```python
from build123d import *

# Parameters (mm, degrees)
SKETCH1_W           = 76.2
SKETCH1_H           = 50.8
SKETCH1_R           = 6.35
BOSS_EXTRUDE1_DEPTH = 3.175
BOSS_EXTRUDE2_DEPTH = 38.1
FILLET1_R           = 3.175
SKETCH3_2_R         = 4.7625
BOSS_EXTRUDE3_DEPTH = 31.75


with BuildPart() as part:
    # Sketch1 → Boss-Extrude1 (new body)
    with BuildSketch(Plane.XY):
        Rectangle(SKETCH1_W, SKETCH1_H)
        with Locations((-25.4, 0)):
            Circle(SKETCH1_R, mode=Mode.SUBTRACT)
        with Locations((25.4, 0)):
            Circle(SKETCH1_R, mode=Mode.SUBTRACT)
    extrude(amount=BOSS_EXTRUDE1_DEPTH)

    # Sketch2 → Boss-Extrude2 (add)
    with BuildSketch(Plane(origin=(0, 0, 0), x_dir=(0, 0, -1), z_dir=(1, 0, 0))):
        with BuildLine():
            Line((0, 38.1), (0, 25.4))
            Line((0, 25.4), (-3.175, 25.4))
            Line((-3.175, 25.4), (-3.175, 31.000484171))
            ThreePointArc((-3.175, 31.000484171), (-18.2200956, 41.988564967), (0, 38.1))
        make_face()
    extrude(amount=-BOSS_EXTRUDE2_DEPTH)

    # Fillet1
    fillet1_edges = [part.edges().sort_by_distance(p)[0] for p in [
        (-19.05, 31.000484171, 3.175),
    ]]
    fillet(fillet1_edges, radius=FILLET1_R)

    # Sketch3<2> → Boss-Extrude3 (add)
    with BuildSketch(Plane(origin=(0, 0, 0), x_dir=(0, 0, -1), z_dir=(1, 0, 0))):
        with Locations((-9.525, 38.1)):
            Circle(SKETCH3_2_R)
    extrude(amount=BOSS_EXTRUDE3_DEPTH)


solid = part.part
```
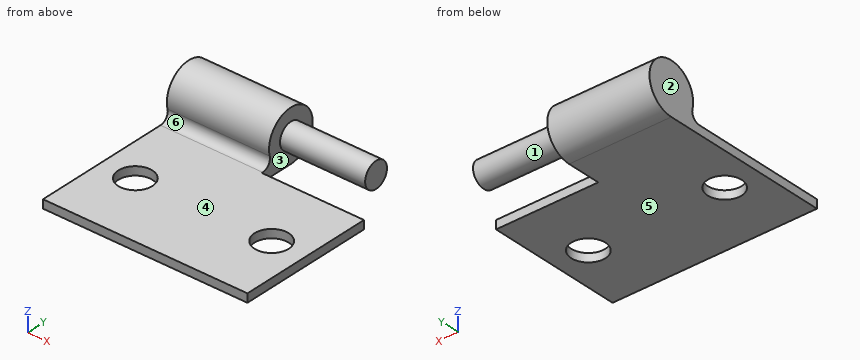
Verification items for the finished model (mm, model axes). Face numbers are marked on the shaded views. A direction names the side the tool comes from. Round coordinates to 2 decimals unless told otherwise and drop trailing zeros. Order: outer loops, then holes, each group sorted by start corner. A loop starts at its lowest first (then second) coordinate and runs counter-clockwise, first axis right, second up. Notation, with made-up numbers: (61, -9) -> (77, -9) arc R34 ccw to (77, 27) -> close; hole circle Ø2 at (-15.5, 60.5). An arc over 180 degrees is marked (long way). Put each result on its own line as item: value. Start each with the question number.
(1) Section check C-C (z = 12.5). Enter the section's corners in (x, y).
(2) Section check D-D (z = 2). Enter the section's corners in (x, y), then the cut area to 3 significant figures.
(3) Section check A-A (y = 0). Enter the section's corners in (x, z) (3 decimals).
(4) Depth check by flat-ended pin: pin 1 Ø4 at (x, z) = (-22.5, 9) entering from -Y (3 decimals); pin 2 Ø10 at (x, z) = (5.5, 13.5) entering from -Y; pin 3 Ø5 at (y, z) = (39.5, 8) entering from +X; pin 4 Ø1 at (x, y) = (-25, 6) entering from -Z. Enter the tip coordinate at first touch or a pass-through.
(5) Section check B-B (x = 23.5). Enter the section's corners in (y, z) (1 decimal).
(6) Tool access check on the marked faces 1 and 2. Record the directions out of +Z, -Z, +X, -X, +Y, -Y that give a thin tool (end or side, any length) a straight path to the whole face; none if there is none.
(7) Material ranges on line 1 along Y through (x, z) = (25.4, 1.85); line 2 along Z through (x, y) = (16.5, -21) (3 decimals); line 3 along Y through (x, z) = (-25.4, 1.1), recorded low to high.
(8) Draft check along Z on the marked faces 3, 4, 5 and 6. Enter one of: +Z half, -Z half, draft (parallel to the pull), parting line (faces both ways), or undercut.
Completed:
1. outline: (-38.1, 29.05) -> (0, 29.05) -> (0, 34.38) -> (31.75, 34.38) -> (31.75, 41.82) -> (0, 41.82) -> (0, 47.15) -> (-38.1, 47.15) -> close
2. outline: (-38.1, -25.4) -> (38.1, -25.4) -> (38.1, 25.4) -> (0, 25.4) -> (0, 43.94) -> (-38.1, 43.94) -> close; hole circle Ø12.7 at (-25.4, 0); hole circle Ø12.7 at (25.4, 0)
2. area: 4,320 mm2
3. outline: (-38.1, 0) -> (-31.75, 0) -> (-31.75, 3.175) -> (-38.1, 3.175) -> close; (-19.05, 0) -> (19.05, 0) -> (19.05, 3.175) -> (-19.05, 3.175) -> close; (31.75, 0) -> (38.1, 0) -> (38.1, 3.175) -> (31.75, 3.175) -> close
4. pin 1: stops at y = 28.575
4. pin 2: stops at y = 33.34
4. pin 3: stops at x = 31.75
4. pin 4: stops at z = 0
5. outline: (-25.4, 0) -> (-6.1, 0) -> (-6.1, 3.2) -> (-25.4, 3.2) -> close; (6.1, 0) -> (25.4, 0) -> (25.4, 3.2) -> (6.1, 3.2) -> close; circle Ø9.5 at (38.1, 9.5)
6. face 1: +X
6. face 2: +Z, -Z, -X, +Y, -Y
7. line 1: y = -25.4 to -6.35, 6.35 to 25.4
7. line 2: z = 0 to 3.175
7. line 3: y = -25.4 to -6.35, 6.35 to 42.54
8. face 3: draft
8. face 4: +Z half
8. face 5: -Z half
8. face 6: undercut
